from build123d import *

# Parameters (mm, degrees)
F0_W     = 1168.4
F0_H     = 355.6
F1_DEPTH = 406.4
F2_W     = 457.2
F2_H     = 177.8
F3_DEPTH = 355.6
F2_W_2   = 317.5
F2_H_2   = 317.5
F4_DEPTH = 317.5


with BuildPart() as f1:
    # F0 (on Top) → F1 (new body)
    with BuildSketch(Plane.XY):
        with Locations((-14.636927, -52.226185)):
            Rectangle(F0_W, F0_H)
    extrude(amount=F1_DEPTH)

    # F2 (on face) → F3 (cut)
    with BuildSketch(Plane.XZ.offset(230.026185)):
        with Locations((213.963073, 317.5)):
            Rectangle(F2_W, F2_H)
    extrude(amount=-F3_DEPTH, mode=Mode.SUBTRACT)

    # F2 (on face) → F4 (cut)
    with BuildSketch(Plane.XZ.offset(230.026185)):
        with Locations((-313.086927, 247.65)):
            Rectangle(F2_W_2, F2_H_2)
    extrude(amount=-F4_DEPTH, mode=Mode.SUBTRACT)


solid = f1.part
Input: part model. Units: mm. Frame: model coordinates. A direction names the side the tool comes from. Coordinates: 2 decimals unless noted, no trailing zeros. Write each loop counter-clockwise with the first axis right and the second up, starting at its lowest first coordinate (ties: lowest second). Pieces come first, ordered by that corner, then holes. Notation, with made-up numbers: M 9.25,-19.5 L 30.25,-19.5 A23 ccw 30.25,-7.5 Z; hole C 34,-31.5 d1. An arc over 180 degrees is marked long. Answer as a JSON object with one key per item and string values. Group by question number.
(1) Set-up query: faces 5 (the face through (-471.837, -73, 245)), 6 (the face through (-311, 108, 406.4)), 7 (the face through (211, -55, 228.6)). Return all of +Z, -Z, +X, -X, +Y, -Y with unobstructed straight access to the full face (end or side cutting, diameter ignored); none if empty.
(2) Section A-A on z = 280.5. Output: boundary loops of the cut face in (x, y).
(3) Section C-C on z = 203. Output: boundary loops of the cut face in (x, y), plus the area to 3 significant figures.
(4) Section D-D on y = 13.5. Output: boundary loops of the cut face in (x, z), plus the area to 3 significant figures.
(5) Section B-B on x = -335. Output: boundary loops of the cut face in (y, z).
(6) Ray query, line 1 along X through (y, z) = (-109, 329.5); line 2 along X through (y, z) = (-101.5, 201); line 3 along Z through (x, y) = (279.5, 10.5). Return the intervals inside material, ascending. Write a range as [from, to].
(7) Mould query, pull axis X, two halves, no side actions, for faces 1 (the face through (569.563, -55, 200)), 2 (the face through (-598.837, -55, 200)), 3 (the face through (505, -50, 406.4)), 4 (the face through (-154.337, -73, 245)). Classes: pulls with the +X half, pulls with the -X half, needs draft (parallel to the pull), parting line crosses it, or undercut.
(8) Contact query for flat-ended pins moving along their axis: P1, Ø10, axis at x = 279.5, y = -157.5, coming from the +Z side; P2, Ø12, axis at x = -370, y = 26, coming from the +Z side. Output: stop coordinate, or through.
Result set:
{
 "1": {"face 5": "+Z, -Y", "face 6": "+Z, +X, -X, +Y, -Y", "face 7": "+Z, +Y, -Y"},
 "2": {"outline": "M -598.84,-230.03 L -471.84,-230.03 L -471.84,87.47 L -154.34,87.47 L -154.34,-230.03 L -14.64,-230.03 L -14.64,125.57 L -598.84,125.57 Z; M 442.56,-230.03 L 569.56,-230.03 L 569.56,125.57 L 442.56,125.57 Z"},
 "3": {"outline": "M -598.84,-230.03 L -471.84,-230.03 L -471.84,87.47 L -154.34,87.47 L -154.34,-230.03 L 569.56,-230.03 L 569.56,125.57 L -598.84,125.57 Z", "area": "315,000 mm2"},
 "4": {"outline": "M -598.84,0 L 569.56,0 L 569.56,406.4 L 442.56,406.4 L 442.56,228.6 L -14.64,228.6 L -14.64,406.4 L -154.34,406.4 L -154.34,88.9 L -471.84,88.9 L -471.84,406.4 L -598.84,406.4 Z", "area": "293,000 mm2"},
 "5": {"outline": "M -230.03,0 L 125.57,0 L 125.57,406.4 L 87.47,406.4 L 87.47,88.9 L -230.03,88.9 Z"},
 "6": {"line 1": "x = [-598.84, -471.84], [-154.34, -14.64], [442.56, 569.56]", "line 2": "x = [-598.84, -471.84], [-154.34, 569.56]", "line 3": "z = [0, 228.6]"},
 "7": {"face 1": "pulls with the +X half", "face 2": "pulls with the -X half", "face 3": "needs draft", "face 4": "undercut"},
 "8": {"P1": "stops at z = 228.6", "P2": "stops at z = 88.9"}
}
